The model under review builds one solid part; all positions refer to its coordinate system, in mm. Round coordinates to 2 decimals unless told otherwise and drop trailing zeros. Write each loop counter-clockwise with the first axis right and the second up, starting at its lowest first coordinate (ties: lowest second). Pieces come first, ordered by that corner, then holes. Notation, with made-up numbers: M -3.75,27.5 L 30.25,27.5 A19 ccw 30.25,44.5 Z; hole C -6.75,26 d10. An arc over 180 degrees is marked long. Write item = value, one per line. Start each with the question number.
Item 1: The part is to be moulded in two halves that separate along Y. For faces 1 (the flat face through (-13, 1, 0)), 2 (the cylindrical face through (-9.665, -2.241, 2.465)), 3 (the flat face through (-1, 55, 2)), say which applies: +Y half, -Y half, draft (parallel to the pull), parting line (faces both ways), or undercut.
Item 2: Take a section at B-B, the plane x = 16. Give the boundary of the cut face in (y, z).
Item 3: Take a section at C-C, the plane y = -47.5. Give the boundary of the cut face in (x, z).
Item 4: To check wall thickness, follow line 1 along Y through (x, z) = (0, 2.9); line 2 along Y through (x, z) = (49.5, 3.9); line 3 along Y through (x, z) = (-16, 2). State the ranges of each line that lie inside material, in increasing order.
Item 5: Take a section at D-D, the plane x = -48. Give the boundary of the cut face in (y, z), plus the area to 3 significant figures.
Item 6: Take a section at A-A, the plane y = 9. Give the boundary of the cut face in (x, z), plus the area to 4 significant figures.
from build123d import *

# Parameters (mm, degrees)
SKETCH_1_W               = 114
SKETCH_1_H               = 110
SKETCH_1_R               = 11.25
EXTRUDE_1_DEPTH          = 5
SKETCH_2_R               = 4
CUT_EXTRUDE_1_DEPTH      = 80.366239674
MIRROR_2_COPY_1_SKETCH_R = 4
MIRROR_2_COPY_1_DEPTH    = 80.366239674
HOLE_WIZARD_M4_2_D       = 3.3
HOLE_WIZARD_M4_3_D       = 3.3
HOLE_WIZARD_M4_4_D       = 3.3
SKETCH_3_R               = 4.5
CUT_EXTRUDE_2_DEPTH      = 80.366239674


with BuildPart() as part:
    # 草图1 → 凸台-拉伸1 (new body)
    with BuildSketch(Plane.XY):
        Rectangle(SKETCH_1_W, SKETCH_1_H)
        with Locations((0, 9)):
            Circle(SKETCH_1_R, mode=Mode.SUBTRACT)
    extrude(amount=EXTRUDE_1_DEPTH)

    # 草图2 → 切除-拉伸1 (cut, through all)
    with BuildSketch(Plane.XY.offset(5)):
        with Locations((-48, 47.5)):
            Circle(SKETCH_2_R)
    cut_extrude_1 = extrude(amount=-CUT_EXTRUDE_1_DEPTH, mode=Mode.SUBTRACT)

    # 镜向1: 切除-拉伸1 across plane
    add(cut_extrude_1.mirror(Plane.ZX), mode=Mode.SUBTRACT)

    # 镜向2: 切除-拉伸1 across plane
    add(cut_extrude_1.mirror(Plane(origin=(0, 0, 0), x_dir=(0, 0, 1), z_dir=(1, 0, 0))), mode=Mode.SUBTRACT)

    # 镜向2 copy 1 sketch → 镜向2 copy 1 (cut, through all)
    with BuildSketch(Plane(origin=(0, 0, 5), x_dir=(-1, 0, 0), z_dir=(0, 0, 1))):
        with Locations((-48, 47.5)):
            Circle(MIRROR_2_COPY_1_SKETCH_R)
    extrude(amount=-MIRROR_2_COPY_1_DEPTH, mode=Mode.SUBTRACT)

    # M4 螺纹孔的螺纹孔钻头2 (through all)
    with Locations(Plane(origin=(-16, 9, 5), x_dir=(1, 0, 0), z_dir=(0, 0, 1))):
        with Locations((0, 0)):
            Hole(HOLE_WIZARD_M4_2_D / 2)

    # M4 螺纹孔的螺纹孔钻头3 (through all)
    with Locations(Plane(origin=(-11.313708499, 20.313708499, 5), x_dir=(1, 0, 0), z_dir=(0, 0, 1))):
        with Locations((0, 0), (0, -22.627416998)):
            Hole(HOLE_WIZARD_M4_3_D / 2)

    # M4 螺纹孔的螺纹孔钻头4 (through all)
    with Locations(Plane(origin=(11.313708499, 20.313708499, 5), x_dir=(1, 0, 0), z_dir=(0, 0, 1))):
        with Locations((0, 0), (4.686291501, -11.313708499), (0, -22.627416998)):
            Hole(HOLE_WIZARD_M4_4_D / 2)

    # 草图3 → 切除-拉伸2 (cut, through all)
    with BuildSketch(Plane.XY.offset(5)):
        with Locations((0, 47.5)):
            Circle(SKETCH_3_R)
    extrude(amount=-CUT_EXTRUDE_2_DEPTH, mode=Mode.SUBTRACT)


solid = part.part
Response values:
q1.face_1 = draft
q1.face_2 = undercut
q1.face_3 = +Y half
q2.outline = M -55,0 L 7.35,0 L 7.35,5 L -55,5 Z; M 10.65,0 L 55,0 L 55,5 L 10.65,5 Z
q3.outline = M -57,0 L -52,0 L -52,5 L -57,5 Z; M -44,0 L 44,0 L 44,5 L -44,5 Z; M 52,0 L 57,0 L 57,5 L 52,5 Z
q4.line_1 = -55 to -2.25, 20.25 to 43, 52 to 55
q4.line_2 = -55 to -51.21, -43.79 to 43.79, 51.21 to 55
q4.line_3 = -55 to 7.35, 10.65 to 55
q5.outline = M -55,0 L -51.5,0 L -51.5,5 L -55,5 Z; M -43.5,0 L 43.5,0 L 43.5,5 L -43.5,5 Z; M 51.5,0 L 55,0 L 55,5 L 51.5,5 Z
q5.area = 470 mm2
q6.outline = M -57,0 L -17.65,0 L -17.65,5 L -57,5 Z; M -14.35,0 L -11.25,0 L -11.25,5 L -14.35,5 Z; M 11.25,0 L 14.35,0 L 14.35,5 L 11.25,5 Z; M 17.65,0 L 57,0 L 57,5 L 17.65,5 Z
q6.area = 424.5 mm2
